```python
from build123d import *

# Parameters (mm, degrees)
SKETCH1_W           = 15
SKETCH1_H           = 15
SKETCH1_W_2         = 11
SKETCH1_H_2         = 11
BOSS_EXTRUDE1_DEPTH = 66
SKETCH3_R           = 1.6
CUT_EXTRUDE1_DEPTH  = 70.32532005
SKETCH4_R           = 1.6
CUT_EXTRUDE2_DEPTH  = 70.32532005


with BuildPart() as part:
    # Sketch1 → Boss-Extrude1 (new body)
    with BuildSketch(Plane(origin=(0, 0, 0), x_dir=(1, 0, 0), z_dir=(0, 1, 0))):
        with Locations((7.5, 7.5)):
            Rectangle(SKETCH1_W, SKETCH1_H)
        with Locations((7.5, 7.5)):
            Rectangle(SKETCH1_W_2, SKETCH1_H_2, mode=Mode.SUBTRACT)
    extrude(amount=BOSS_EXTRUDE1_DEPTH)

    # Sketch3 → Cut-Extrude1 (cut, through all)
    with BuildSketch(Plane(origin=(0, 0, -15), x_dir=(-1, 0, 0), z_dir=(0, 0, -1))):
        with Locations((-7.5, 21)):
            Circle(SKETCH3_R)
        with Locations((-7.5, 45)):
            Circle(SKETCH3_R)
    extrude(amount=-CUT_EXTRUDE1_DEPTH, mode=Mode.SUBTRACT)

    # Sketch4 → Cut-Extrude2 (cut, through all)
    with BuildSketch(Plane.ZY):
        with Locations((-7.5, 13)):
            Circle(SKETCH4_R)
        with Locations((-7.5, 29)):
            Circle(SKETCH4_R)
    extrude(amount=-CUT_EXTRUDE2_DEPTH, mode=Mode.SUBTRACT)


solid = part.part
```
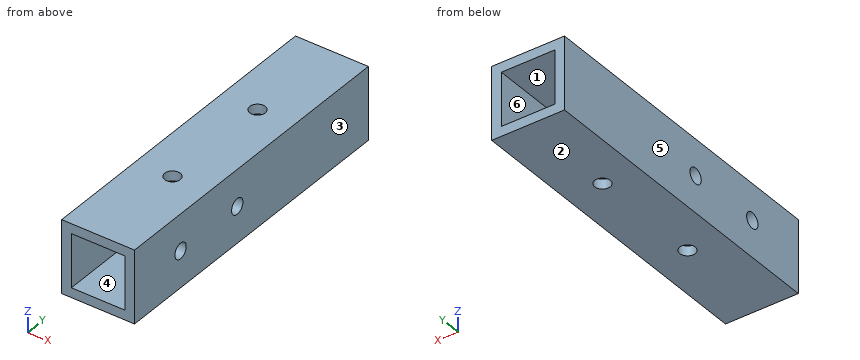
Source: CAD feature listing. Evaluate the final solid. Frame: model axes, mm. Face numbers are marked on the shaded views. A direction names the side the tool comes from. Coordinates: 2 decimals unless noted, no trailing zeros. Loops run counter-clockwise (first coordinate to the right, second up) from the corner with the lowest first, then second, coordinate; pieces in that order, holes last. Notation, with made-up numbers: M 78.5,47 L 126.5,47 A22 ccw 126.5,71 Z; hole C -9.75,47.25 d8. An arc over 180 degrees is marked long. Use CSV: the item, a comma, the result in double quotes.
(1) Line query: line 1 (Y direction, x = 7.5, z = -1.4); line 2 (X direction, y = 62.5, z = -10); line 3 (Y direction, x = 1.05, z = -7.5). Output: solid intervals per line, ascending. Write a range as [from, to].
Answers follow:
line 1,"[0, 19.4], [22.6, 43.4], [46.6, 66]"
line 2,"[0, 2], [13, 15]"
line 3,"[0, 11.4], [14.6, 27.4], [30.6, 66]"
(2) Cut plane A-A on z = -7.5. Return loops of the section in (x, y), and give its area (3 significant figures).
Answers follow:
outline,"M 0,0 L 2,0 L 2,11.4 L 0,11.4 Z; M 0,14.6 L 2,14.6 L 2,27.4 L 0,27.4 Z; M 0,30.6 L 2,30.6 L 2,66 L 0,66 Z; M 13,0 L 15,0 L 15,11.4 L 13,11.4 Z; M 13,14.6 L 15,14.6 L 15,27.4 L 13,27.4 Z; M 13,30.6 L 15,30.6 L 15,66 L 13,66 Z"
area,"238 mm²"
(3) Reachability of the marked faces 5 and 6 from +Z, -Z, +X, -X, +Y, -Y: full face, straight path, thin tool, end or side. Return the list, or none.
Answers follow:
face 5,"+Z, -Z, -X, +Y, -Y"
face 6,"+Y, -Y"
(4) Draft query along X for the marked faces 1, 2, 3 and 4. Return one class per face: pulls with the +X half, pulls with the -X half, needs draft (parallel to the pull), parting line crosses it, or undercut.
Answers follow:
face 1,"undercut"
face 2,"needs draft"
face 3,"pulls with the +X half"
face 4,"undercut"
(5) Cut plane D-D on z = -10.25. Return loops of the section in (x, y).
Answers follow:
outline,"M 0,0 L 2,0 L 2,66 L 0,66 Z; M 13,0 L 15,0 L 15,66 L 13,66 Z"
(6) Cut plane B-B on y = 13. Return loops of the section in (x, z).
Answers follow:
outline,"M 0,-15 L 15,-15 L 15,-9.1 L 13,-9.1 L 13,-13 L 2,-13 L 2,-9.1 L 0,-9.1 Z; M 0,-5.9 L 2,-5.9 L 2,-2 L 13,-2 L 13,-5.9 L 15,-5.9 L 15,0 L 0,0 Z"
(7) Cut plane C-C on x = 11. Return loops of the section in (y, z).
Answers follow:
outline,"M 0,-15 L 66,-15 L 66,-13 L 0,-13 Z; M 0,-2 L 66,-2 L 66,0 L 0,0 Z"
